Autodesk Inventor part; units mm, degrees
ref_plane "YZ Plane" through (0, 0, 0) normal (1, 0, 0) x (0, 1, 0)
ref_plane "XZ Plane" through (0, 0, 0) normal (0, 1, 0) x (-1, 0, 0)
ref_plane "XY Plane" through (0, 0, 0) normal (0, 0, 1) x (1, 0, 0)
sketch "スケッチ1" plane through (0, 0, 0) normal (0, 0, 1) x (1, 0, 0)
  line L0 (0, 0) -> (140, 0)
  line L1 (140, 0) -> (140, 100)
  line L2 (140, 100) -> (0, 100)
  line L3 (0, 100) -> (0, 0)
  dimension "d0" = 140
  dimension "d1" = 100
extrude "押し出し1" add sketch "スケッチ1" along normal blind 2
sketch "スケッチ2" plane through (0, 0, 2) normal (0, 0, 1) x (1, 0, 0)
  line L0 (140, 100) -> (0, 100)
  line L1 (70, 100) -> (70, 0) construction
  line L2 (0, 0) -> (140, 0)
  line L3 (2.5, 85) -> (5, 85)
  line L4 (5, 83) -> (5, 17)
  line L5 (5, 15) -> (2.5, 15)
  line L6 (2.5, 17) -> (2.5, 83)
  line L7 (0, 100) -> (0, 0)
  line L8 (0, 50) -> (140, 50) construction
  line L9 (140, 0) -> (140, 100)
  arc A0 (2.5, 85) -> (2.5, 83) centre (2.5, 84) ccw
  arc A1 (5, 83) -> (5, 85) centre (5, 84) ccw
  arc A2 (2.5, 17) -> (2.5, 15) centre (2.5, 16) ccw
  arc A3 (5, 15) -> (5, 17) centre (5, 16) ccw
  line L10 (137.5, 85) -> (135, 85)
  line L11 (135, 83) -> (135, 17)
  line L12 (135, 15) -> (137.5, 15)
  line L13 (137.5, 17) -> (137.5, 83)
  line L14 (140, 50) -> (0, 50) construction
  arc A4 (137.5, 83) -> (137.5, 85) centre (137.5, 84) ccw
  arc A5 (135, 85) -> (135, 83) centre (135, 84) ccw
  arc A6 (137.5, 15) -> (137.5, 17) centre (137.5, 16) ccw
  arc A7 (135, 17) -> (135, 15) centre (135, 16) ccw
  dimension "d4" = 2.5
  dimension "d5" = 2.5
  dimension "d6" = 70
  dimension "d7" = 2
  dimension "d8" = 2
  dimension "d9" = 2
  dimension "d10" = 2
extrude "押し出し2" cut sketch "スケッチ2" against normal through all contours L3 A1 L4 A3 L5 A2 L6 A0 | A4 L13 A6 L12 A7 L11 A5 L10
sketch "スケッチ3" plane through (0, 0, 2) normal (0, 0, 1) x (1, 0, 0)
  line L0 (140, 100) -> (0, 100)
  line L1 (70, 100) -> (70, 0) construction
  line L2 (0, 0) -> (140, 0)
  point P0 (70, 80)
  dimension "d13" = 20
hole "穴1" at (70, 80, 2) direction (0, 0, -1) diameter 22 end through all
properties part number "body_top"
Input: part model. Units: mm. Frame: model coordinates. Give positions to 0.01 mm unless a question says otherwise; leave off trailing zeros. Order: outer loops, then holes, each group sorted by start corner. A loop starts at its lowest first (then second) coordinate and runs counter-clockwise, first axis right, second up. Notation, with made-up numbers: (55.25, -23.75) - (65.25, -23.75) arc R28 cw to (65.25, 10.25) - close; hole circle Ø3 at (-39, 21). An arc over 180 degrees is marked (long way). Answer as a JSON object with one key per item and string values. Group by question number.
Q1. Cut plane A-A, the plane x = 70. Output: boundary loops of the cut face in (y, z), then the cut area to 3 significant figures.
Q2. Line query: probe 1 along X at (y, z) = (57, 0.6); probe 2 along X at (y, z) = (80, 1.4); probe 3 along Y at (x, z) = (70, 0.6). Output: solid intervals per line, ascending.
Q3. Cut plane D-D, the plane y = 51.5. Output: boundary loops of the cut face in (x, z).
Q4. Cut plane B-B, the plane y = 80. Output: boundary loops of the cut face in (x, z), then the cut area to 3 significant figures.
Q5. Mould query, pull axis X, two halves, no side actions, for faces 1 (the face through (70, 91, 1)), 2 (the face through (69, 51, 0)). Classes: pulls with the +X half, pulls with the -X half, needs draft (parallel to the pull), parting line crosses it, or undercut.
Q6. Cut plane C-C, the plane z = 0.35. Output: boundary loops of the cut face in (x, y), then the cut area to 3 significant figures.
Results:
{
 "1": {"outline": "(0, 0) - (69, 0) - (69, 2) - (0, 2) - close; (91, 0) - (100, 0) - (100, 2) - (91, 2) - close", "area": "156 mm^2"},
 "2": {"probe 1": "0 to 2.5, 5 to 135, 137.5 to 140", "probe 2": "0 to 2.5, 5 to 59, 81 to 135, 137.5 to 140", "probe 3": "0 to 69, 91 to 100"},
 "3": {"outline": "(0, 0) - (2.5, 0) - (2.5, 2) - (0, 2) - close; (5, 0) - (135, 0) - (135, 2) - (5, 2) - close; (137.5, 0) - (140, 0) - (140, 2) - (137.5, 2) - close"},
 "4": {"outline": "(0, 0) - (2.5, 0) - (2.5, 2) - (0, 2) - close; (5, 0) - (59, 0) - (59, 2) - (5, 2) - close; (81, 0) - (135, 0) - (135, 2) - (81, 2) - close; (137.5, 0) - (140, 0) - (140, 2) - (137.5, 2) - close", "area": "226 mm^2"},
 "5": {"face 1": "undercut", "face 2": "needs draft"},
 "6": {"outline": "(0, 0) - (140, 0) - (140, 100) - (0, 100) - close; hole (2.5, 15) - (5, 15) arc R1 ccw to (5, 17) - (5, 83) arc R1 ccw to (5, 85) - (2.5, 85) arc R1 ccw to (2.5, 83) - (2.5, 17) arc R1 ccw to start; hole circle Ø22 at (70, 80); hole (135, 15) - (137.5, 15) arc R1 ccw to (137.5, 17) - (137.5, 83) arc R1 ccw to (137.5, 85) - (135, 85) arc R1 ccw to (135, 83) - (135, 17) arc R1 ccw to start", "area": "13,300 mm^2"}
}
